Work out the finished part from the listing and answer in its coordinate system (mm). A direction names the side the tool comes from. Coordinates: 2 decimals unless noted, no trailing zeros. Loops run counter-clockwise (first coordinate to the right, second up) from the corner with the lowest first, then second, coordinate; pieces in that order, holes last.
```python
from build123d import *

# Parameters (mm, degrees)
F2_SIZE2 = 1
F2_SIZE  = 18
F4_DEPTH = 2.5


with BuildPart() as f1:
    # F0 (on Front) → F1 (revolve)
    with BuildSketch(Plane.XZ):
        with BuildLine():
            Line((0, -40), (0, 0))
            ThreePointArc((0, 0), (-3.146824, -0.486346), (-6, -1.9))
            Line((-6, -1.9), (-6, -2.7))
            Line((-6, -2.7), (-1.5, -2.7))
            Line((-1.5, -2.7), (-1.5, -40))
            Line((-1.5, -40), (0, -40))
        make_face()
    revolve(axis=Axis((0, 0, -20), (0, 0, -1)))

    # F2
    f2_edges = [f1.edges().sort_by_distance(p)[0] for p in [
        (1.5, 0, -40),
    ]]
    chamfer(f2_edges, length=F2_SIZE, length2=F2_SIZE2)

    # F3 (on Top) → F4 (cut)
    with BuildSketch(Plane.XY):
        Polygon((1.010363, -1.75), (2.020726, 0), (1.010363, 1.75), (-1.010363, 1.75), (-2.020726, 0), (-1.010363, -1.75), align=None)
    extrude(amount=-F4_DEPTH, mode=Mode.SUBTRACT)


solid = f1.part
```
1. Straight lines are drawn through the part: probe 1 along X at (y, z) = (-0.25, -18); probe 2 along X at (y, z) = (3.25, -2); probe 3 along Z at (x, y) = (5, 0.5). For each, find the intervals that lie inside material, in ascending order.
2. A cutting plane is placed at A-A, the plane z = -23. Give the vertices of the cut face in (x, y), then the cut area to 3 significant figures.
3. A cutting plane is placed at B-B, the plane z = -4.5. Give the vertices of the cut face in (x, y), then the cut area to 3 significant figures.
4. For faces 1 (the flat face through (-1.5, 0.9, -1.3)), 2 (the flat face through (0, 0, -40)), 3 (the flat face through (-1.2, -1.2, -2.7)), determine the directions among +Z, -Z, +X, -X, +Y, -Y from which every point of the face is accessible in a straight line to the end or side of a thin tool.
5. Each of these flat-tipped pins is pushed along its axis until it touches: P1, Ø1.5, axis at x = 0, y = -3.5, coming from the +Z side; P2, Ø4, axis at y = -3, z = -25.5, coming from the +X side; P3, Ø4, axis at y = 0, z = -12, coming from the +X side. Where does it stop, or does it pass through?
Answers below:
1. probe 1: x = -1.48 to 1.48
1. probe 2: x = -5.04 to 5.04
1. probe 3: z = -2.7 to -1.29
2. outline: circle Ø2.89 at (0, 0)
2. area: 6.55 mm2
3. outline: circle Ø3 at (0, 0)
3. area: 7.07 mm2
4. face 1: +Z
4. face 2: -Z, +X, -X, +Y, -Y
4. face 3: -Z
5. P1: stops at z = -0.37
5. P2: stops at x = 0.85
5. P3: stops at x = 1.5
